```python
from build123d import *

# Parameters (mm, degrees)
SKETCH3_R             = 1.9812
BOSS_EXTRUDE1_DEPTH   = 7.7978
BOSS_EXTRUDE1_2_DEPTH = 7.7978
BOSS_EXTRUDE2_DEPTH   = 1.6002


with BuildPart() as part:
    # Sketch3 → Boss-Extrude1 (new body, symmetric)
    with BuildSketch(Plane.XY):
        with Locations((-5.9944, 0)):
            Circle(SKETCH3_R)
    extrude(amount=BOSS_EXTRUDE1_DEPTH, both=True)



with BuildPart() as body_2:
    # Sketch3 → Boss-Extrude1 2 (new body, symmetric)
    with BuildSketch(Plane.XY):
        with Locations((5.9944, 0)):
            Circle(SKETCH3_R)
    extrude(amount=BOSS_EXTRUDE1_2_DEPTH, both=True)


with BuildPart() as part_1:
    add(part.part)

    add(body_2.part)  # Boss-Extrude2 merges body 2
    # Sketch4 → Boss-Extrude2 (add)
    with BuildSketch(Plane.XY.offset(7.0358)):
        with BuildLine():
            ThreePointArc((-3.908114, 4.991761), (-11.4046, 0), (-3.908114, -4.991761))
            ThreePointArc((-3.908114, -4.991761), (0, -4.207923), (3.908114, -4.991761))
            ThreePointArc((3.908114, -4.991761), (11.4046, 0), (3.908114, 4.991761))
            ThreePointArc((3.908114, 4.991761), (0, 4.207923), (-3.908114, 4.991761))
        make_face()
    boss_extrude2 = extrude(amount=-BOSS_EXTRUDE2_DEPTH)

    # Mirror1: Boss-Extrude2 across plane
    add(boss_extrude2.mirror(Plane.XY))

    # Sketch5 → Cut-Revolve1 (revolve, cut)
    with BuildSketch(Plane(origin=(0, 0, 0), x_dir=(1, 0, 0), z_dir=(0, 1, 0))):
        with BuildLine():
            Line((-5.9944, 7.7978), (-5.9944, 7.1374))
            ThreePointArc((-5.9944, 7.1374), (-4.950216, 7.306848), (-4.0132, 7.7978))
            Line((-4.0132, 7.7978), (-5.9944, 7.7978))
        make_face()
        with BuildLine():
            Line((-5.9944, -7.1374), (-5.9944, -7.7978))
            Line((-5.9944, -7.7978), (-4.0132, -7.7978))
            ThreePointArc((-4.0132, -7.7978), (-4.950216, -7.306848), (-5.9944, -7.1374))
        make_face()
    cut_revolve1 = revolve(axis=Axis((-5.9944, 0, 7.7978), (0, 0, -1)), mode=Mode.SUBTRACT)

    # Mirror2: Cut-Revolve1 across plane
    add(cut_revolve1.mirror(Plane(origin=(0, 0, 0), x_dir=(0, 0, 1), z_dir=(1, 0, 0))), mode=Mode.SUBTRACT)


solid = part_1.part
```
Read the model definition and answer for the solid it produces. Units are mm, in the model's axes. A direction names the side the tool comes from. Give positions to 0.01 mm unless a question says otherwise; leave off trailing zeros. Order: outer loops, then holes, each group sorted by start corner. A loop starts at its lowest first (then second) coordinate and runs counter-clockwise, first axis right, second up. Notation, with made-up numbers: (-32, 73) -> (8, 73) arc R29 ccw to (8, 103) -> close; hole circle Ø3 at (87, 55). An arc over 180 degrees is marked (long way). One line per item, written item: value. Start each with the question number.
(1) The part is cut by section A-A (x = -1.75). Determine the outline of the cut face in (y, z), and give its area (3 significant figures).
(2) For a pull along Z with two mould halves and no side action, classify faces 4 (the flat face through (0, 0, 5.436)), 5 (the flat face through (0, 0, 7.036)), 6 (the cylindrical face through (7.884, 0.595, -7.411)) as released by +Z, released by -Z, zero draft, split by the parting line, or undercut.
(3) A tool of negligible diameter and unlimited length cuts with its end or side. For faces 1 (the cylindrical face through (7.884, 0.595, 7.422)), 2 (the cylindrical face through (-4.105, 0.595, 0.076)), 3 (the flat face through (0, 0, -7.036)), from which of +Z, -Z, +X, -X, +Y, -Y can it reach the whole face along a straight path? Write none if from no direction.
(4) Flat-ended cylindrical pins translate along their axes: P1, Ø1, axis at x = 9, y = -4, coming from the +Z side; P2, Ø3, axis at y = 0, z = -1.5, coming from the -X side; P3, Ø3, axis at x = 3.5, y = 2.5, coming from the -Z side. Find the tip coordinate at first contact, or state that the pin passes through.
(5) Straight lines are drawn through the part: L1, parallel to Z at x = -4, y = -1.5; L2, parallel to Y at x = 6, z = 2.25; L3, parallel to Y at x = 5, z = 4.25. For each, find the intervals that lie inside material, in ascending order.
(6) The part is cut by section B-B (y = -4.5). Determine the outline of the cut face in (x, z), and give its area (3 significant figures).
(7) The part is cut by section D-D (y = -2.5). Determine the outline of the cut face in (x, z).
(8) The part is cut by section C-C (z = 2). Determine the outline of the cut face in (x, y), and give its area (3 significant figures).
Taken from the geometry:
1. outline: (-4.36, -7.04) -> (4.36, -7.04) -> (4.36, -5.44) -> (-4.36, -5.44) -> close; (-4.36, 5.44) -> (4.36, 5.44) -> (4.36, 7.04) -> (-4.36, 7.04) -> close
1. area: 27.9 mm^2
2. face 4: undercut
2. face 5: released by +Z
2. face 6: zero draft
3. face 1: +Z
3. face 2: none
3. face 3: -Z
4. P1: z = 7.04
4. P2: x = -7.98
4. P3: z = -7.04
5. L1: -7.04 to -5.44, 5.44 to 7.04
5. L2: -1.98 to 1.98
5. L3: -1.71 to 1.71
6. outline: (-9, -7.04) -> (-2.42, -7.04) -> (-2.42, -5.44) -> (-9, -5.44) -> close; (-9, 5.44) -> (-2.42, 5.44) -> (-2.42, 7.04) -> (-9, 7.04) -> close; (2.42, -7.04) -> (9, -7.04) -> (9, -5.44) -> (2.42, -5.44) -> close; (2.42, 5.44) -> (9, 5.44) -> (9, 7.04) -> (2.42, 7.04) -> close
6. area: 42.1 mm^2
7. outline: (-10.79, -7.04) -> (10.79, -7.04) -> (10.79, -5.44) -> (-10.79, -5.44) -> close; (-10.79, 5.44) -> (10.79, 5.44) -> (10.79, 7.04) -> (-10.79, 7.04) -> close
8. outline: circle Ø3.96 at (-5.99, 0); circle Ø3.96 at (5.99, 0)
8. area: 24.7 mm^2
